Verification items for this drawing (mm, ordinates from the low corner). Coordinates: 2 decimals unless noted, no trailing zeros. Order: outer loops, then holes, each group sorted by start corner. A loop starts at its lowest first (then second) coordinate and runs counter-clockwise, first axis right, second up. Notation, with made-up numbers: (65, -21.5) -> (113, -21.5) arc R11 ccw to (113, -12.5) -> close; hole circle Ø8 at (85, 7.5). An arc over 180 degrees is marked (long way). Write item = value, one per line. Start each with the question number.
1. Thickness scan on line 1 along Z through (x, y) = (74.5, 6.5); line 2 along Z through (x, y) = (76.5, 42); line 3 along Y through (x, z) = (128, 7). Record the ranges inside material, lowest first. Write a range as from..to.
2. Cross-section at B-B on y = 6. Record the cut outline in (x, z), plus the area to 3 significant figures.
3. Cross-section at A-A on x = 118. Record the cut outline in (y, z), plus the area to 3 significant figures.
4. Go/stop test with flat-tipped pins: P1, Ø4, axis at x = 120.5, y = 41, coming from the -Z side; P2, Ø4, axis at x = 136.5, z = 65, coming from the -Y side. Record where each tip stops, or that it passes through.
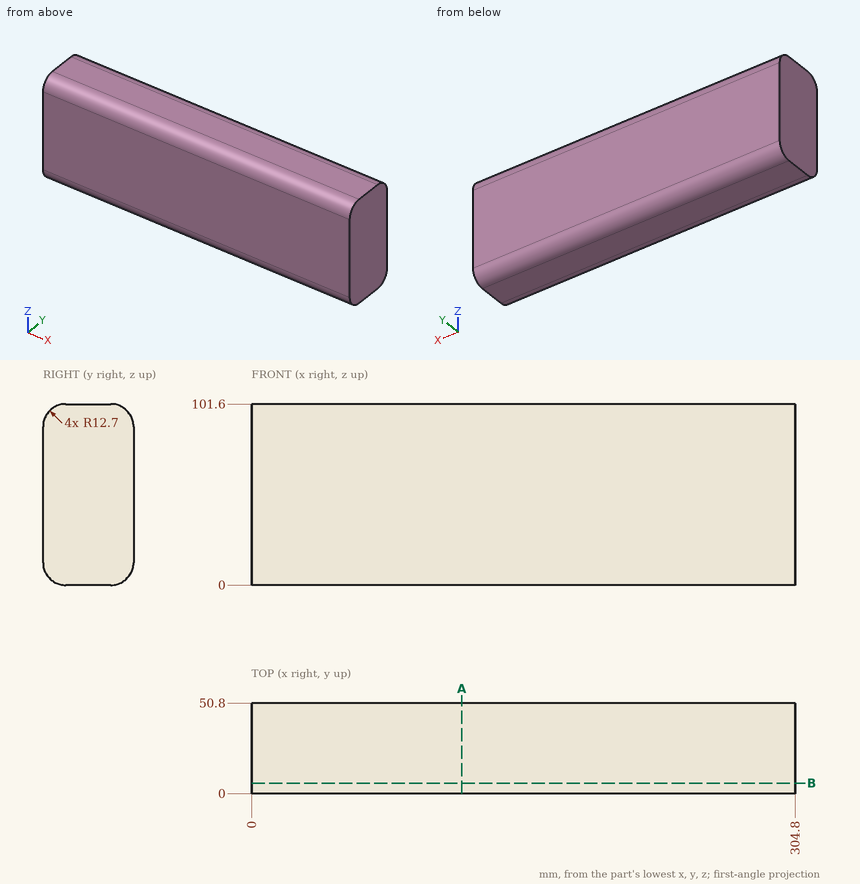
Worked out:
q1.line_1 = 1.62..99.98
q1.line_2 = 0.61..100.99
q1.line_3 = 1.35..49.45
q2.outline = (0, 1.91) -> (304.8, 1.91) -> (304.8, 99.69) -> (0, 99.69) -> close
q2.area = 29,800 mm²
q3.outline = (0, 12.7) arc R12.7 ccw to (12.7, 0) -> (38.1, 0) arc R12.7 ccw to (50.8, 12.7) -> (50.8, 88.9) arc R12.7 ccw to (38.1, 101.6) -> (12.7, 101.6) arc R12.7 ccw to (0, 88.9) -> close
q3.area = 5,020 mm²
q4.P1 = 0.03
q4.P2 = 0
